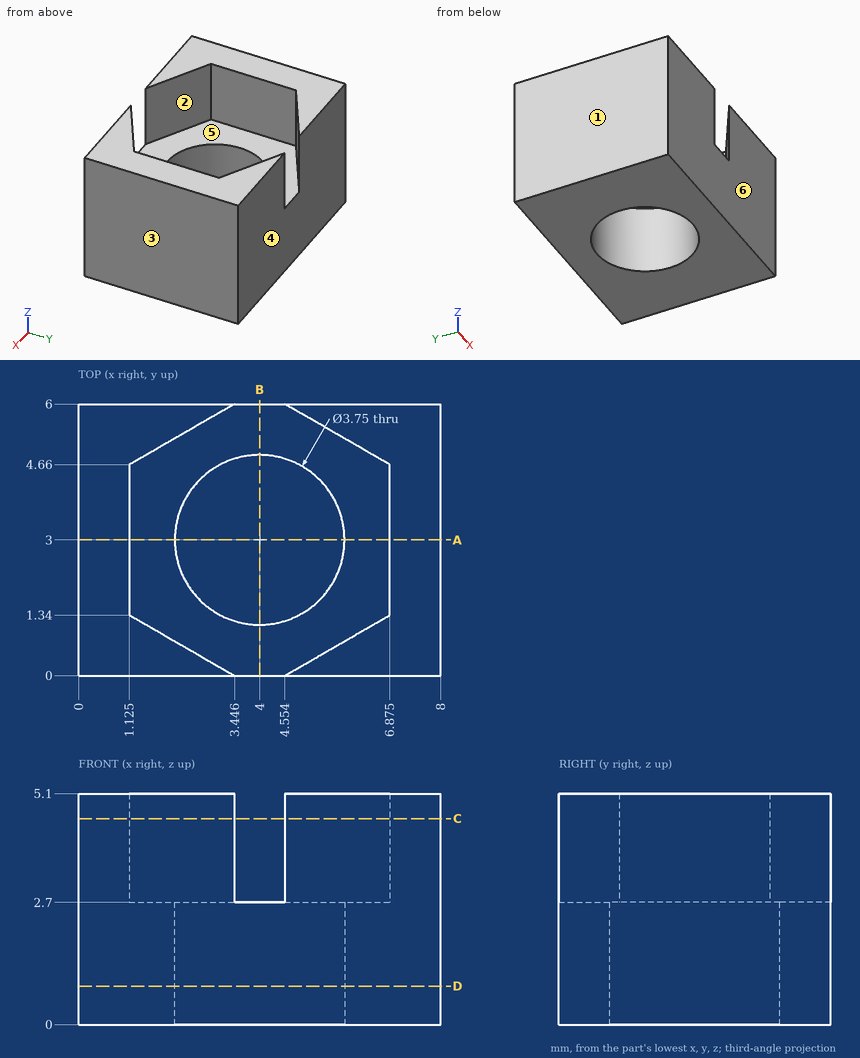
Print and shaded views of the part. All mm, measured from the part's lowest x, y and z. A direction names the side the tool comes from. Round coordinates to 2 decimals unless told otherwise and drop trailing zeros. Write each loop counter-clockwise with the first axis right and the second up, starting at its lowest first coordinate (ties: lowest second). Pieces come first, ordered by that corner, then holes.
(1) Slice it at D-D, the plane z = 0.85. Write the cut outline in (x, y) (3 decimals).
(2) 3-axis set-ups, long thin cutter, end or side, ignore diameter. For the marked faces 1 and 2: which of +Z, -Z, +X, -X, +Y, -Y reach the whole face in a straight line?
(3) Probe line 1 along Y through (x, z) = (4, 1.2) (3 decimals); line 2 along X through (y, z) = (3.25, 4.35) (3 decimals); line 3 along Z through (x, y) = (3.5, 0.5). List the from-to ranges inside material, lowest first.
(4) Drop flat-ended pins along their axis: P1, Ø2, axis at x = 4, y = 3, coming from the -Z side; P2, Ø3, axis at y = 2, z = 1.5, coming from the -X side. Give the stop position or say it passes through.
(5) Mould opens along Y. For the marked faces 3, 4, 5 and 6 say: pulls with the +Y half, pulls with the -Y half, needs draft (parallel to the pull), parting line crosses it, or undercut.
(6) Slice it at C-C, the plane z = 4.55. Write the cut outline in (x, y) (3 decimals).
(7) Slice it at A-A, the plane y = 3. Write the cut outline in (x, z) (3 decimals), and give its area (3 significant figures).
(8) Slice it at B-B, the plane x = 4. Write the cut outline in (y, z) (3 decimals).
From the geometry:
1. outline: (0, 0) - (8, 0) - (8, 6) - (0, 6) - close; hole circle Ø3.75 at (4, 3)
2. face 1: +Z, -Z, -X, +Y, -Y
2. face 2: +Z
3. line 1: y = 0 to 1.125, 4.875 to 6
3. line 2: x = 0 to 1.125, 6.875 to 8
3. line 3: z = 0 to 2.7
4. P1: passes through
4. P2: stops at x = 0
5. face 3: needs draft
5. face 4: pulls with the +Y half
5. face 5: undercut
5. face 6: pulls with the -Y half
6. outline: (0, 0) - (3.446, 0) - (1.125, 1.34) - (1.125, 4.66) - (3.446, 6) - (0, 6) - close; (4.554, 0) - (8, 0) - (8, 6) - (4.554, 6) - (6.875, 4.66) - (6.875, 1.34) - close
7. outline: (0, 0) - (2.125, 0) - (2.125, 2.7) - (1.125, 2.7) - (1.125, 5.1) - (0, 5.1) - close; (5.875, 0) - (8, 0) - (8, 5.1) - (6.875, 5.1) - (6.875, 2.7) - (5.875, 2.7) - close
7. area: 16.9 mm2
8. outline: (0, 0) - (1.125, 0) - (1.125, 2.7) - (0, 2.7) - close; (4.875, 0) - (6, 0) - (6, 2.7) - (4.875, 2.7) - close
